Source: CAD feature listing. Evaluate the final solid. Frame: model axes, mm. A direction names the side the tool comes from. Give positions to 0.01 mm unless a question says otherwise; leave off trailing zeros. Loops run counter-clockwise (first coordinate to the right, second up) from the corner with the lowest first, then second, coordinate; pieces in that order, holes last.
from build123d import *

# Parameters (mm, degrees)
BOX013_W      = 637
BOX013_H      = 15
BOX013_DEPTH  = 20
BOX012_W      = 637
BOX012_H      = 15
BOX012_DEPTH  = 20
SKETCH012_R   = 2.05
HOLE007_DEPTH = 1291.481784


with BuildPart() as cube008:
    # Box013 → Box013 (new body)
    with BuildSketch(Plane(origin=(1.5, 1.5, -1.5), x_dir=(1, 0, 0), z_dir=(0, 0, 1))):
        with Locations((318.5, 7.5)):
            Rectangle(BOX013_W, BOX013_H)
    extrude(amount=BOX013_DEPTH)


with BuildPart() as top_front_body:
    # Box012 → Box012 (new body)
    with BuildSketch(Plane(origin=(1.5, 0, 0), x_dir=(1, 0, 0), z_dir=(0, 0, 1))):
        with Locations((318.5, 7.5)):
            Rectangle(BOX012_W, BOX012_H)
    extrude(amount=BOX012_DEPTH)

    # Cut: cut Cube008
    add(cube008.part, mode=Mode.SUBTRACT)


with BuildPart() as top_front_body_1:
    # Cut placement: moved
    add(top_front_body.part.moved(Location((0, 1.5, 250))))


with BuildPart() as top_front_body_2:
    # BaseFeature005 placement: moved
    add(top_front_body_1.part.moved(Location((0, -1.5, -250))))

    # Sketch012 → Hole007 (cut, through all)
    with BuildSketch(Plane.XZ.offset(1.5)):
        with Locations((-7.75, 9.25)):
            Circle(SKETCH012_R)
    hole007 = extrude(amount=-HOLE007_DEPTH, mode=Mode.SUBTRACT)

    # Mirrored004: Hole007 across Sketch012 Axis0
    add(hole007.mirror(Plane(origin=(320, -1.5, 19.25), x_dir=(0, -1, 0), z_dir=(1, 0, 0))), mode=Mode.SUBTRACT)


with BuildPart() as top_front_body_3:
    # Body005 placement: moved
    add(top_front_body_2.part.moved(Location((0, 1.5, 260))))


solid = top_front_body_3.part
1) Cut plane A-A (x = 306). Return loops of the section in (y, z), and give its area (4 significant figures).
Checks:
outline: (1.5, 260) - (3, 260) - (3, 278.5) - (16.5, 278.5) - (16.5, 280) - (1.5, 280) - close
area: 50.25 mm2
2) Contact query for flat-ended pins moving along their axis: P1, Ø5, axis at x = 455.5, y = 15, coming from the -Z side; P2, Ø8, axis at x = 462.5, z = 275, coming from the +Y side. Output: stop coordinate, or through.
Checks:
P1: stops at z = 278.5
P2: stops at y = 16.5
3) Pull-direction query (X, two-part tool) for faces 1 (the flat face through (1.5, 2, 274)), 2 (the flat face through (316, 1.5, 270)), 3 (the flat face through (638.5, 2, 274)); classes: released by +X, released by -X, zero draft, split by the parting line, or undercut.
Checks:
face 1: released by -X
face 2: zero draft
face 3: released by +X
4) Cut plane B-B (y = 11.75). Return loops of the section in (x, z), and give its area (4 significant figures).
Checks:
outline: (1.5, 278.5) - (638.5, 278.5) - (638.5, 280) - (1.5, 280) - close
area: 955.5 mm2
5) Ray query, probe 1 along Z at (x, y) = (389.5, 11.25); probe 2 along Y at (x, z) = (603, 266). Return the intervals inside material, ascending.
Checks:
probe 1: z = 278.5 to 280
probe 2: y = 1.5 to 3
6) Reachability of faces 4 (the flat face through (316, 9, 280)), 5 (the flat face through (316, 10, 278.5)) from +Z, -Z, +X, -X, +Y, -Y: full face, straight path, thin tool, end or side. Return the list, or none.
Checks:
face 4: +Z, +X, -X, +Y, -Y
face 5: -Z, +X, -X, +Y
7) Cut plane C-C (z = 269.5). Return loops of the section in (x, y), and give its area (4 significant figures).
Checks:
outline: (1.5, 1.5) - (638.5, 1.5) - (638.5, 3) - (1.5, 3) - close
area: 955.5 mm2
